from build123d import *

# Parameters (mm, degrees)
EXTRUDE_1_DEPTH     = 112
EXTRUDE_START       = -2.25
EXTRUDE_2_DEPTH     = 3
SKETCH_9_W          = 6
SKETCH_9_H          = 99
CUT_EXTRUDE_3_DEPTH = 10
SKETCH_10_W         = 225.5
SKETCH_10_H         = 7
EXTRUDE_3_DEPTH     = 2
SKETCH_5_R          = 1.5
CUT_EXTRUDE_2_DEPTH = 2
CUT_EXTRUDE_4_DEPTH = 4


with BuildPart() as part:
    # 草图1 → 凸台-拉伸1 (new, symmetric)
    with BuildSketch(Plane.XY):
        Polygon((11.28405341, 15.648913828), (3.47340992, 15.648913828), (3.47340992, 20.648913828), (-56.981135534, 96.648913828), (-58.71594659, 96.648913828), (-58.71594659, 103.648913828), align=None)
    extrude(amount=EXTRUDE_1_DEPTH, both=True)

    # 草图8 → 凸台-拉伸2 (add)
    with BuildSketch(Plane(origin=(0, 0, -112), x_dir=(-1, 0, 0), z_dir=(0, 0, -1)).offset(EXTRUDE_START)):
        Polygon((-3.47340992, 15.648913828), (-11.28405341, 15.648913828), (-11.28405341, 26.893468065), (49.77141481, 103.648913828), (58.71594659, 103.648913828), (58.71594659, 96.648913828), (56.981135534, 96.648913828), (-3.47340992, 20.648913828), align=None)
    extrude_2 = extrude(amount=EXTRUDE_2_DEPTH)

    # 镜向1: 凸台-拉伸2 across plane
    add(extrude_2.mirror(Plane.XY))

    # 草图9 → 切除-拉伸3 (cut)
    with BuildSketch(Plane(origin=(14.535037867, 11.561961939, 0), x_dir=(0, 0, -1), z_dir=(0.7826010541756485, 0.6225235658215388, 0))):
        with Locations((12, 59.722267293)):
            Rectangle(SKETCH_9_W, SKETCH_9_H)
        with Locations((0, 59.722267293)):
            Rectangle(SKETCH_9_W, SKETCH_9_H)
        with Locations((24, 59.722267293)):
            Rectangle(SKETCH_9_W, SKETCH_9_H)
        with Locations((36, 59.722267293)):
            Rectangle(SKETCH_9_W, SKETCH_9_H)
        with Locations((48, 59.722267293)):
            Rectangle(SKETCH_9_W, SKETCH_9_H)
        with Locations((60, 59.722267293)):
            Rectangle(SKETCH_9_W, SKETCH_9_H)
        with Locations((72, 59.722267293)):
            Rectangle(SKETCH_9_W, SKETCH_9_H)
        with Locations((84, 59.722267293)):
            Rectangle(SKETCH_9_W, SKETCH_9_H)
        with Locations((96, 59.722267293)):
            Rectangle(SKETCH_9_W, SKETCH_9_H)
        with Locations((-12, 59.722267293)):
            Rectangle(SKETCH_9_W, SKETCH_9_H)
        with Locations((-24, 59.722267293)):
            Rectangle(SKETCH_9_W, SKETCH_9_H)
        with Locations((-36, 59.722267293)):
            Rectangle(SKETCH_9_W, SKETCH_9_H)
        with Locations((-48, 59.722267293)):
            Rectangle(SKETCH_9_W, SKETCH_9_H)
        with Locations((-60, 59.722267293)):
            Rectangle(SKETCH_9_W, SKETCH_9_H)
        with Locations((-72, 59.722267293)):
            Rectangle(SKETCH_9_W, SKETCH_9_H)
        with Locations((-84, 59.722267293)):
            Rectangle(SKETCH_9_W, SKETCH_9_H)
        with Locations((-96, 59.722267293)):
            Rectangle(SKETCH_9_W, SKETCH_9_H)
    extrude(amount=-CUT_EXTRUDE_3_DEPTH, mode=Mode.SUBTRACT)

    # 草图10 → 凸台-拉伸3 (add)
    with BuildSketch(Plane.ZY.offset(58.71594659)):
        with Locations((0, 100.148913828)):
            Rectangle(SKETCH_10_W, SKETCH_10_H)
    extrude(amount=EXTRUDE_3_DEPTH)

    # 草图5 → 切除-拉伸2 (cut)
    with BuildSketch(Plane.XZ.offset(-96.648913828)):
        with Locations(Location((-58.71594659, -86.5, 0), (0, 0, 270))):
            Circle(SKETCH_5_R)
        with Locations(Location((-58.71594659, 86.5, 0), (0, 0, 270))):
            Circle(SKETCH_5_R)
    extrude(amount=-CUT_EXTRUDE_2_DEPTH, mode=Mode.SUBTRACT)

    # 草图12 → 切除-拉伸4 (cut)
    with BuildSketch(Plane.XY.offset(112.75)):
        Polygon((-60.71594659, 103.648913828), (-60.71594659, 96.597994862), (-56.981135534, 96.648913828), (-44.624218302, 81.114503593), (-44.624218302, 97.178152504), (-49.77141481, 103.648913828), align=None)
    cut_extrude_4 = extrude(amount=-CUT_EXTRUDE_4_DEPTH, mode=Mode.SUBTRACT)

    # 镜向2: 切除-拉伸4 across plane
    add(cut_extrude_4.mirror(Plane.XY), mode=Mode.SUBTRACT)


solid = part.part
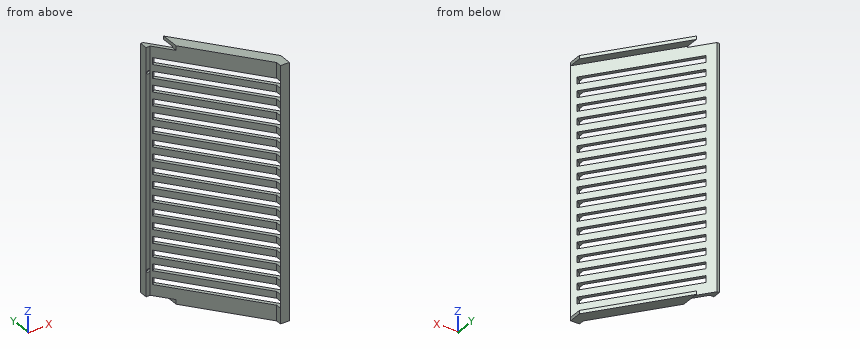
Check sheet for the modelled part. Datum: model origin and axes. Units: mm. Round coordinates to 2 decimals unless told otherwise and drop trailing zeros.
1. Scan lines: probe 1 along Z at (x, y) = (-3.5, 40.5); probe 2 along X at (y, z) = (97, 86); probe 3 along X at (y, z) = (97.65, -86.5). Record each from-to range of solid material in increasing order.
2. Gauge pin test, flat ends, axial feed: pin 1 Ø1.8 at (x, z) = (-58.72, -86.5) entering from -Y; pin 2 Ø13 at (x, y) = (-50, 90) entering from -Z; pin 3 Ø4 at (y, z) = (75, 8.5) entering from +X; pin 4 Ø6 at (y, z) = (31, -40.5) entering from +X. Record the tip position at first contact, or that the pin passes through.
3. Sectioned sample at A-A on x = -11. Give the number of separate pieces and of enclosed holes in the cut face, and give its area (3 significant figures).
Recorded:
1. probe 1: z = -112.75 to -109.75, 109.75 to 112.75
1. probe 2: x = -60.72 to -60.13, -57.3 to -53.51
1. probe 3: x = -60.72 to -60.22, -57.22 to -53.94
2. pin 1: stops at y = 98.65
2. pin 2: stops at z = -112.75
2. pin 3: stops at x = -34.34
2. pin 4: stops at x = 1.46
3. separate pieces: 18
3. enclosed holes: 0
3. area: 663 mm2
